The listing builds one solid part. Answer for the finished solid, in the listing's coordinates (mm). A direction names the side the tool comes from. Round coordinates to 2 decimals unless told otherwise and drop trailing zeros. Loops run counter-clockwise (first coordinate to the right, second up) from the corner with the lowest first, then second, coordinate; pieces in that order, holes last. Notation, with made-up numbers: (-27, 17.25) -> (19, 17.25) arc R36 cw to (19, 56.25) -> close; hole circle Ø10 at (1, 89.25). An arc over 180 degrees is marked (long way). One line per question, with ' | ' between items.
Autodesk Inventor part; units mm, degrees
ref_plane "YZ Plane" through (0, 0, 0) normal (1, 0, 0) x (0, 1, 0)
ref_plane "XZ Plane" through (0, 0, 0) normal (0, 1, 0) x (-1, 0, 0)
ref_plane "XY Plane" through (0, 0, 0) normal (0, 0, 1) x (1, 0, 0)
sketch "Sketch1" plane through (0, 0, 0) normal (0, 0, 1) x (1, 0, 0)
  circle A0 centre (0, 0) radius 1.0033
  circle A1 centre (0, 0) radius 3.175
  line L0 (-1.905, -8.255) -> (1.905, -8.255)
  line L1 (1.905, -8.255) -> (1.905, -2.54)
  line L2 (-1.905, -8.255) -> (-1.905, -2.54)
  circle A2 centre (0, -6.35) radius 1.0033
  line L3 (1.905, -8.255) -> (3.81, -8.255)
  line L4 (3.81, -8.255) -> (1.905, -2.54)
  line L5 (-1.905, -8.255) -> (-3.81, -8.255)
  line L6 (-3.81, -8.255) -> (-1.905, -2.54)
  point P0 (0, -8.255)
  dimension "d0" = 2.0066
  dimension "d1" = 6.35
  dimension "d2" = 3.81
  dimension "d3" = 2.0066
  dimension "d4" = 5.715
  dimension "d5" = 1.905
  dimension "d10" = 1.905
  dimension "d11" = 1.905
extrude "Extrusion1" add sketch "Sketch1" along normal blind 5.08 contours A1 | A1 L1 L0 L2
extrude "Extrusion3" add sketch "Sketch1" along normal blind 5.08 contours L2 L5 L6 | L4 L3 L1
fillet "Fillet1" radius 1.5875 4 edges at (3.81, -8.255, 2.54) (-3.81, -8.255, 2.54) (1.905, -2.54, 2.54) (-1.905, -2.54, 2.54)
Q1. A cutting plane is placed at A-A on x = 0. Give the vertices of the cut face in (y, z) (3 decimals).
Numbers:
outline: (-8.255, 0) -> (-7.353, 0) -> (-7.353, 5.08) -> (-8.255, 5.08) -> close; (-5.347, 0) -> (-1.003, 0) -> (-1.003, 5.08) -> (-5.347, 5.08) -> close; (1.003, 0) -> (3.175, 0) -> (3.175, 5.08) -> (1.003, 5.08) -> close
Q2. Find the intervals of material crossed by line 1 (Y direction, x = 0, z = 4.7) (3 decimals); line 2 (X direction, y = -7.25, z = 1.7); line 3 (X direction, y = -0.5, z = 3.1), in increasing order. Write a range as from..to.
Numbers:
line 1: -8.255..-7.353, -5.347..-1.003, 1.003..3.175 | line 2: -3.08..-0.44, 0.44..3.08 | line 3: -3.14..-0.87, 0.87..3.14
Q3. A cutting plane is placed at C-C on z = 1.3. Give the number of separate pieces and of enclosed holes in the cut face, plus the area to 3 significant figures.
Numbers:
separate pieces: 1 | enclosed holes: 2 | area: 54.4 mm^2
Q4. For a pull along Y with two mould halves and no side action, classify faces 1 (the face through (-0.74, -0.68, 2.5)), 2 (the face through (0, -8.255, 3)), 3 (the face through (0, -2, 5.08)) as pulls with the +Y half, pulls with the -Y half, needs draft (parallel to the pull), parting line crosses it, or undercut.
Numbers:
face 1: undercut | face 2: pulls with the -Y half | face 3: needs draft
Q5. A cutting plane is placed at B-B on y = 0. Give the vertices of the cut face in (x, z) (3 decimals), plus the area to 3 significant figures.
Numbers:
outline: (-3.175, 0) -> (-1.003, 0) -> (-1.003, 5.08) -> (-3.175, 5.08) -> close; (1.003, 0) -> (3.175, 0) -> (3.175, 5.08) -> (1.003, 5.08) -> close | area: 22.1 mm^2
Q6. For faces 4 (the face through (-2.67, -4.84, 2.5)), 5 (the face through (2.67, -4.84, 2.5)), 6 (the face through (-0.22, -5.37, 2.5)), determine the directions among +Z, -Z, +X, -X, +Y, -Y from which every point of the face is accessible in a straight line to the end or side of a thin tool.
Numbers:
face 4: +Z, -Z, -X | face 5: +Z, -Z, +X | face 6: +Z, -Z
Q7. Given pin 1 Ø1.5 at (y, z) = (-2, 1.5) entering from -X; pin 2 Ø2 at (x, z) = (-2, 2) entering from +Y, each flat-ended and moving along its own axis, determine where each tip first touches the part or whether it passes through.
Numbers:
pin 1: x = -2.92 | pin 2: y = 3.01
Q8. A cutting plane is placed at D-D on y = -5.75. Give the vertices of the cut face in (x, z) (3 decimals), plus the area to 3 significant figures.
Numbers:
outline: (-2.975, 0) -> (-0.804, 0) -> (-0.804, 5.08) -> (-2.975, 5.08) -> close; (0.804, 0) -> (2.975, 0) -> (2.975, 5.08) -> (0.804, 5.08) -> close | area: 22.1 mm^2
